from build123d import *

# Parameters (mm, degrees)
SKETCH_R     = 60
PAD_DEPTH    = 2
SKETCH001_R  = 20
PAD001_DEPTH = 2
PAD002_DEPTH = 6.5
SKETCH003_R  = 4.5
PAD003_DEPTH = 2
FILLET_R     = 1
SKETCH004_R  = 2
POCKET_DEPTH = 12.501


with BuildPart() as part:
    # Sketch → Pad (new body)
    with BuildSketch(Plane.XY):
        Circle(SKETCH_R)
    extrude(amount=PAD_DEPTH)

    # Sketch001 (on Face3 of Pad) → Pad001 (join)
    with BuildSketch(Plane.XY.offset(2)):
        Circle(SKETCH001_R)
    extrude(amount=PAD001_DEPTH)

    # Sketch002 (on Face5 of Pad001) → Pad002 (join)
    with BuildSketch(Plane.XY.offset(4)):
        Polygon((4.907477, 8.5), (-4.907477, 8.5), (-9.814955, 0), (-4.907477, -8.5), (4.907477, -8.5), (9.814955, 0), align=None)
    extrude(amount=PAD002_DEPTH)

    # Sketch003 (on Face12 of Pad002) → Pad003 (join)
    with BuildSketch(Plane.XY.offset(10.5)):
        Circle(SKETCH003_R)
    extrude(amount=PAD003_DEPTH)

    # Fillet
    fillet_edges = [part.edges().sort_by_distance(p)[0] for p in [
        (-4.5, 0, 12.5),
    ]]
    fillet(fillet_edges, radius=FILLET_R)

    # Sketch004 (on Face4 of Fillet) → Pocket (cut, through all)
    with BuildSketch(Plane.XY.offset(12.5)):
        Circle(SKETCH004_R)
    extrude(amount=-POCKET_DEPTH, mode=Mode.SUBTRACT)


solid = part.part
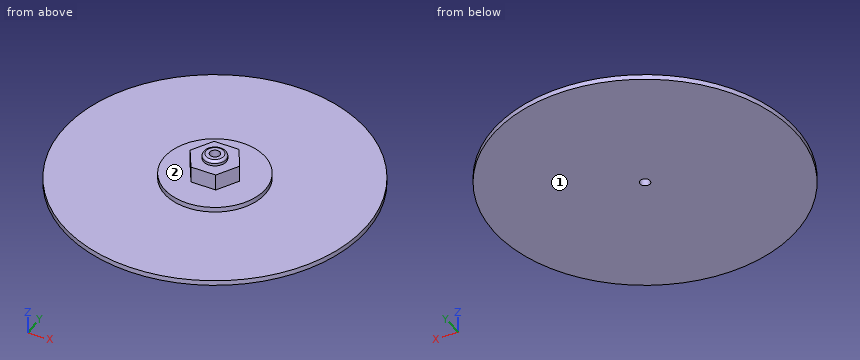
Can you work these out from the model? Positions are in its coordinate system, mm. Face numbers are marked on the shaded views. A direction names the side the tool comes from. Round coordinates to 2 decimals unless told otherwise and drop trailing zeros. Write each loop counter-clockwise with the first axis right and the second up, starting at its lowest first coordinate (ties: lowest second). Pieces come first, ordered by that corner, then holes. Notation, with made-up numbers: (47, -36) - (105, -36) arc R31 cw to (105, -11) - close; hole circle Ø8 at (19, 13). An arc over 180 degrees is marked (long way). Write each question's results on one line, items separated by ' | '. Start each with the question number.
1) For pin 1 Ø8 at (x, y) = (33, 32.5) entering from +Z; pin 2 Ø2 at (y, z) = (-21, 5) entering from -X; pin 3 Ø2 at (x, z) = (0, 8.5) entering from +Y; pin 4 Ø3 at (x, z) = (0, 7) entering from -Y, each with a flat end and sliding along its axis, tell me the tip position at first contact or that it passes through.
2) Suppose I cut it at B-B (z = 9). List the corners of the cut face in (x, y) for me.
3) Which directions (+Z, -Z, +X, -X, +Y, -Y) give clear straight access to the entire face, cutting with the end or side of a thin tool? Please do the marked faces 1 and 2.
4) Please list where these lines run through material, in increasing order: line 1 (Y direction, x = 0, z = 9); line 2 (Y direction, x = 0, z = 2.5); line 3 (Z direction, x = 20.5, y = 54).
5) Suppose I cut it at A-A (x = 0). List the corners of the cut face in (y, z) for me, and give its area (3 significant figures).
6) Suppose I cut it at D-D (y = -48.5). List the corners of the cut face in (x, z) for me, and give its area (3 significant figures).
7) Suppose I cut it at C-C (x = 16). List the corners of the cut face in (y, z) for me, and give its area (3 significant figures).
Here are the results:
1) pin 1: stops at z = 2 | pin 2: passes through | pin 3: stops at y = 8.5 | pin 4: stops at y = -8.5
2) outline: (-9.81, 0) - (-4.91, -8.5) - (4.91, -8.5) - (9.81, 0) - (4.91, 8.5) - (-4.91, 8.5) - close; hole circle Ø4 at (0, 0)
3) face 1: -Z, +X, -X, +Y, -Y | face 2: +Z
4) line 1: y = -8.5 to -2, 2 to 8.5 | line 2: y = -20 to -2, 2 to 20 | line 3: z = 0 to 2
5) outline: (-60, 0) - (-2, 0) - (-2, 12.5) - (-3.5, 12.5) arc R1 ccw to (-4.5, 11.5) - (-4.5, 10.5) - (-8.5, 10.5) - (-8.5, 4) - (-20, 4) - (-20, 2) - (-60, 2) - close; (2, 0) - (60, 0) - (60, 2) - (20, 2) - (20, 4) - (8.5, 4) - (8.5, 10.5) - (4.5, 10.5) - (4.5, 11.5) arc R1 ccw to (3.5, 12.5) - (2, 12.5) - close | area: 398 mm2
6) outline: (-35.32, 0) - (35.32, 0) - (35.32, 2) - (-35.32, 2) - close | area: 141 mm2
7) outline: (-57.83, 0) - (57.83, 0) - (57.83, 2) - (12, 2) - (12, 4) - (-12, 4) - (-12, 2) - (-57.83, 2) - close | area: 279 mm2
